Input: part model. Units: mm. Frame: model coordinates. Coordinates: 2 decimals unless noted, no trailing zeros. Order: outer loops, then holes, each group sorted by start corner. A loop starts at its lowest first (then second) coordinate and runs counter-clockwise, first axis right, second up. Notation, with made-up numbers: M 85,-24.5 L 135,-24.5 A8 cw 135,-14.5 Z; hole C 84,60.25 d11. An arc over 180 degrees is marked long. One line per item, written item: value.
```python
from build123d import *

# Parameters (mm, degrees)
SKETCH1_W           = 100
SKETCH1_H           = 20
BOSS_EXTRUDE1_DEPTH = 10
SKETCH2_R           = 2.75
CUT_EXTRUDE1_DEPTH  = 11


with BuildPart() as part:
    # Sketch1 → Boss-Extrude1 (new body)
    with BuildSketch(Plane.XY.offset(10)):
        with Locations((50, 10)):
            Rectangle(SKETCH1_W, SKETCH1_H)
    extrude(amount=-BOSS_EXTRUDE1_DEPTH)

    # Sketch2 → Cut-Extrude1 (cut, through all)
    with BuildSketch(Plane.XY.offset(10)):
        with Locations((94, 10)):
            Circle(SKETCH2_R)
        with Locations((6, 10)):
            Circle(SKETCH2_R)
    extrude(amount=-CUT_EXTRUDE1_DEPTH, mode=Mode.SUBTRACT)


solid = part.part
```
(1) Cut plane D-D on x = 93. Output: boundary loops of the cut face in (y, z).
Data:
outline: M 0,0 L 7.44,0 L 7.44,10 L 0,10 Z; M 12.56,0 L 20,0 L 20,10 L 12.56,10 Z
(2) Cut plane A-A on x = 6. Output: boundary loops of the cut face in (y, z).
Data:
outline: M 0,0 L 7.25,0 L 7.25,10 L 0,10 Z; M 12.75,0 L 20,0 L 20,10 L 12.75,10 Z
(3) Cut plane C-C on z = 8.5. Output: boundary loops of the cut face in (x, y).
Data:
outline: M 0,0 L 100,0 L 100,20 L 0,20 Z; hole C 6,10 d5.5; hole C 94,10 d5.5
(4) First-contact query: pin 1 (5 mm diameter, centred on x = 6, y = 10, fed in from +Z); pin 2 (7 mm diameter, centred on x = 94, y = 10, fed in from -Z). Flat tips, straight axial feed; report the tip coordinate or a pass-through.
Data:
pin 1: passes through
pin 2: stops at z = 0
(5) Draft query along Y for faces 1 (the flat face through (100, 10, 5)), 2 (the cylindrical face through (7.48, 12.32, 5.07)), 3 (the flat face through (49, 0, 5)). Return one class per face: released by +Y, released by -Y, zero draft, split by the parting line, or undercut.
Data:
face 1: zero draft
face 2: undercut
face 3: released by -Y
(6) Cut plane B-B on y = 10. Output: boundary loops of the cut face in (x, z), plus the area to 3 significant figures.
Data:
outline: M 0,0 L 3.25,0 L 3.25,10 L 0,10 Z; M 8.75,0 L 91.25,0 L 91.25,10 L 8.75,10 Z; M 96.75,0 L 100,0 L 100,10 L 96.75,10 Z
area: 890 mm2
(7) Ray query, line 1 (X direction, y = 9.75, z = 1.25); line 2 (Y direction, x = 94, z = 2.5); line 3 (X direction, y = 8.5, z = 6). Return the intervals inside material, ascending. Write a range as from..to.
Data:
line 1: x = 0..3.26, 8.74..91.26, 96.74..100
line 2: y = 0..7.25, 12.75..20
line 3: x = 0..3.7, 8.3..91.7, 96.3..100
